```python
from build123d import *

# Parameters (mm, degrees)
F0_R      = 46.355
F1_DEPTH  = 22.86
F2_R      = 44.1325
F3_DEPTH  = 11.43
F4_R      = 38.1
F5_DEPTH  = 17.78
F6_W      = 81.28
F6_H      = 12.192
F7_DEPTH  = 17.78
F8_R      = 5.715
F9_DEPTH  = 22.861
F10_R     = 1.27
F11_DEPTH = 46.356
F12_W     = 17.272
F12_H     = 8.89
F13_DEPTH = 46.356
F14_R     = 1.6256
F15_DEPTH = 22.861
F16_SIZE  = 1.905
F17_W     = 4.445
F17_H     = 11.43
F18_DEPTH = 46.356
F19_SIZE  = 1.27


with BuildPart() as f1:
    # F0 (on Top) → F1 (new body)
    with BuildSketch(Plane.XY):
        Circle(F0_R)
    extrude(amount=-F1_DEPTH)

    # F2 (on face) → F3 (cut)
    with BuildSketch(Plane.XY):
        Circle(F2_R)
    extrude(amount=-F3_DEPTH, mode=Mode.SUBTRACT)

    # F4 (on Top) → F5 (cut)
    with BuildSketch(Plane.XY):
        Circle(F4_R)
    extrude(amount=-F5_DEPTH, mode=Mode.SUBTRACT)

    # F6 (on Top) → F7 (cut)
    with BuildSketch(Plane.XY):
        Rectangle(F6_W, F6_H)
    extrude(amount=-F7_DEPTH, mode=Mode.SUBTRACT)

    # F8 (on Top) → F9 (cut, through all)
    with BuildSketch(Plane.XY):
        with Locations((-33.782, 0)):
            Circle(F8_R)
        with Locations((33.782, 0)):
            Circle(F8_R)
    extrude(amount=-F9_DEPTH, mode=Mode.SUBTRACT)

    # F10 (on Front) → F11 (cut, through all)
    with BuildSketch(Plane.XZ):
        with Locations((0, -5.842)):
            Circle(F10_R)
    extrude(amount=F11_DEPTH, mode=Mode.SUBTRACT)

    # F12 (on Front) → F13 (cut, through all)
    with BuildSketch(Plane.XZ):
        with Locations((0, -4.445)):
            Rectangle(F12_W, F12_H)
    extrude(amount=-F13_DEPTH, mode=Mode.SUBTRACT)

    # F14 (on Top) → F15 (cut, through all)
    with BuildSketch(Plane.XY):
        with Locations((0, 25.4)):
            Circle(F14_R)
        with Locations((0, -25.4)):
            Circle(F14_R)
    extrude(amount=-F15_DEPTH, mode=Mode.SUBTRACT)

    # F16
    f16_edges = [f1.edges().sort_by_distance(p)[0] for p in [
        (-1.6256, 25.4, -17.78),
        (-1.6256, -25.4, -17.78),
    ]]
    chamfer(f16_edges, length=F16_SIZE)

    # F17 (on Right) → F18 (cut, through all)
    with BuildSketch(Plane.YZ):
        with Locations((15.24, -5.715)):
            Rectangle(F17_W, F17_H)
    extrude(amount=-F18_DEPTH, mode=Mode.SUBTRACT)

    # F19
    f19_edges = [f1.edges().sort_by_distance(p)[0] for p in [
        (-43.771316, 15.259683, -11.43),
    ]]
    chamfer(f19_edges, length=F19_SIZE)


solid = f1.part
```
Geometry: final body of the model. Coordinates: model frame, mm. A direction names the side the tool comes from. Round coordinates to 2 decimals unless told otherwise and drop trailing zeros. Write each loop counter-clockwise with the first axis right and the second up, starting at its lowest first coordinate (ties: lowest second). Pieces come first, ordered by that corner, then holes. Notation, with made-up numbers: (48.25, 14.25) -> (99.25, 14.25) arc R13 cw to (99.25, 31.25) -> close; hole circle Ø4 at (71, -34.75). An arc over 180 degrees is marked (long way). Use CSV: the item, a comma, the result in double quotes. Start each with the question number.
Q1. Section B-B (y = 0). Return loops of the section in (x, z) (1 decimal), plus the area to 3 significant figures.
Q2. Pull-direction query (X, two-part tool) for faces 4 (the face through (-1, 1, -17.78)), 5 (the face through (-10.049, -45.253, -11.27)), 6 (the face through (-42, 17.462, -6)); classes: pulls with the +X half, pulls with the -X half, needs draft (parallel to the pull), parting line crosses it, or undercut.
Q3. First-contact query: pin 1 Ø1.5 at (y, z) = (-13.5, -8) entering from -X; pin 2 Ø2.5 at (x, z) = (39, -14) entering from +Y; pin 3 Ø0.9 at (x, z) = (39.5, -16) entering from -Y. Flat tips, straight axial feed; report the tip coordinate or a pass-through.
Q4. Line query: L1, parallel to Y at x = 0, z = -20.25 (3 decimals); L2, parallel to Z at x = 28.5, y = 26; L3, parallel to Y at x = 8, z = -13.75. Output: solid intervals per line, ascending.
Q5. Section D-D (y = 25.4). Return loops of the section in (x, z) (3 decimals), plus the area to 3 significant figures.
Q6. Section A-A (x = 0). Return loops of the section in (y, z) (1 decimal).
Q7. Reachability of faces 1 (the face through (39.23, 1.72, -20.28)), 2 (the face through (8.636, 44, -5)), 3 (the face through (0.752, 38.093, -14.561)) from +Z, -Z, +X, -X, +Y, -Y: full face, straight path, thin tool, end or side. Return the list, or none.
Q8. Section C-C (x = -35). Return loops of the section in (y, z), plus the area to 3 significant figures.
Result sheet:
1,outline,"(-46.4, -22.9) -> (-39.5, -22.9) -> (-39.5, -17.8) -> (-40.6, -17.8) -> (-40.6, -11.4) -> (-44.1, -11.4) -> (-44.1, 0) -> (-46.4, 0) -> close; (-28.1, -22.9) -> (28.1, -22.9) -> (28.1, -17.8) -> (-28.1, -17.8) -> close; (39.5, -22.9) -> (46.4, -22.9) -> (46.4, 0) -> (44.1, 0) -> (44.1, -11.4) -> (40.6, -11.4) -> (40.6, -17.8) -> (39.5, -17.8) -> close"
1,area,"478 mm²"
2,face 4,"undercut"
2,face 5,"parting line crosses it"
2,face 6,"needs draft"
3,pin 1,"x = -44.57"
3,pin 2,"y = 26.9"
3,pin 3,"y = -24.98"
4,L1,"-46.355 to -27.026, -23.774 to 23.774, 27.026 to 46.355"
4,L2,"-22.86 to -11.43"
4,L3,"-45.66 to -37.25, 37.25 to 45.66"
5,outline,"(-38.777, -22.86) -> (-1.626, -22.86) -> (-1.626, -19.685) -> (-3.531, -17.78) -> (-28.398, -17.78) -> (-28.398, -11.43) -> (-36.09, -11.43) -> (-36.09, 0) -> (-38.777, 0) -> close; (1.626, -22.86) -> (38.777, -22.86) -> (38.777, 0) -> (36.09, 0) -> (36.09, -11.43) -> (28.398, -11.43) -> (28.398, -17.78) -> (3.531, -17.78) -> (1.626, -19.685) -> close"
5,area,"567 mm²"
6,outline,"(-46.4, -22.9) -> (-27, -22.9) -> (-27, -19.7) -> (-28.9, -17.8) -> (-38.1, -17.8) -> (-38.1, -11.4) -> (-44.1, -11.4) -> (-44.1, -7.1) -> (-46.4, -7.1) -> close; (-46.4, -4.6) -> (-44.1, -4.6) -> (-44.1, 0) -> (-46.4, 0) -> close; (-23.8, -22.9) -> (23.8, -22.9) -> (23.8, -19.7) -> (21.9, -17.8) -> (-21.9, -17.8) -> (-23.8, -19.7) -> close; (27, -22.9) -> (46.4, -22.9) -> (46.4, -8.9) -> (44.1, -8.9) -> (44.1, -11.4) -> (38.1, -11.4) -> (38.1, -17.8) -> (28.9, -17.8) -> (27, -19.7) -> close"
7,face 1,"+Z, -Z"
7,face 2,"+Z, +Y"
7,face 3,"+Z"
8,outline,"(-30.39, -22.86) -> (-5.58, -22.86) -> (-5.58, -17.78) -> (-15.05, -17.78) -> (-15.05, -11.43) -> (-26.88, -11.43) -> (-26.88, 0) -> (-30.39, 0) -> close; (5.58, -22.86) -> (30.39, -22.86) -> (30.39, 0) -> (26.88, 0) -> (26.88, -11.43) -> (15.05, -11.43) -> (15.05, -17.78) -> (5.58, -17.78) -> close"
8,area,"527 mm²"
